Geometry check sheet. Reference: the model listing, model coordinates, mm. Face numbers are marked on the shaded views. A direction names the side the tool comes from. Coordinates: 2 decimals unless noted, no trailing zeros. Write each loop counter-clockwise with the first axis right and the second up, starting at its lowest first coordinate (ties: lowest second). Pieces come first, ordered by that corner, then holes.
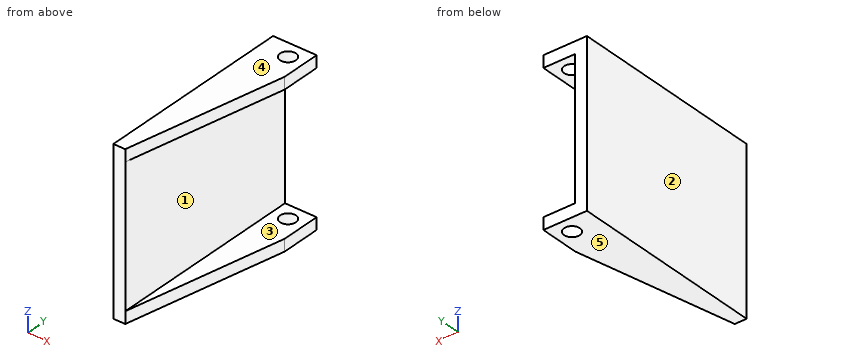
from build123d import *

# Parameters (mm, degrees)
SKETCH1_W           = 40.99099099
SKETCH1_H           = 50
BOSS_EXTRUDE1_DEPTH = 3
BOSS_EXTRUDE3_DEPTH = 3
SKETCH4_R           = 2
CUT_EXTRUDE1_DEPTH  = 3


with BuildPart() as part:
    # Sketch1 → Boss-Extrude1 (new body)
    with BuildSketch(Plane(origin=(0, 0, 0), x_dir=(0, 0, -1), z_dir=(1, 0, 0))):
        Rectangle(SKETCH1_W, SKETCH1_H)
    extrude(amount=BOSS_EXTRUDE1_DEPTH)

    # Sketch3 → Boss-Extrude3 (add)
    with BuildSketch(Plane.XY.offset(20.495495495)):
        Polygon((3, 25), (11, 25), (11, 15), (3, -25), align=None)
    boss_extrude3 = extrude(amount=-BOSS_EXTRUDE3_DEPTH)

    # Sketch4 → Cut-Extrude1 (cut)
    with BuildSketch(Plane.XY.offset(20.495495495)):
        with Locations((7, 21)):
            Circle(SKETCH4_R)
    cut_extrude1 = extrude(amount=-CUT_EXTRUDE1_DEPTH, mode=Mode.SUBTRACT)

    # Mirror1: Boss-Extrude3, Cut-Extrude1 across plane
    add(boss_extrude3.mirror(Plane.XY))
    add(cut_extrude1.mirror(Plane.XY), mode=Mode.SUBTRACT)


solid = part.part
1. Sectioned sample at D-D, the plane x = 10.25. Record the boundary of the cut face in (y, z), and give its area (3 significant figures).
Computed values:
outline: (11.25, -20.5) - (25, -20.5) - (25, -17.5) - (11.25, -17.5) - close; (11.25, 17.5) - (25, 17.5) - (25, 20.5) - (11.25, 20.5) - close
area: 82.5 mm2
2. Draft check along Z on the marked faces 3, 4 and 5. Enter one of: released by +Z, released by -Z, zero draft, split by the parting line, or undercut.
Computed values:
face 3: undercut
face 4: released by +Z
face 5: released by -Z
3. Thickness scan on line 1 along Z through (x, y) = (3.25, 15.5); line 2 along X through (y, z) = (-15, -10.5); line 3 along X through (y, z) = (11, 18.5). Record the ranges inside material, lowest first.
Computed values:
line 1: z = -20.5 to -17.5, 17.5 to 20.5
line 2: x = 0 to 3
line 3: x = 0 to 10.2
4. Gauge pin test, flat ends, axial feed: pin 1 Ø8 at (y, z) = (1.5, 13) entering from +X; pin 2 Ø1 at (x, z) = (9, -16) entering from +Y; pin 3 Ø6.5 at (x, y) = (9, 0) entering from +Z. Record the tip position at first contact, or that the pin passes through.
Computed values:
pin 1: stops at x = 3
pin 2: passes through
pin 3: stops at z = 20.5
5. Sectioned sample at B-B, the plane y = 21. Record the boundary of the cut face in (x, z), and give its area (3 significant figures).
Computed values:
outline: (0, -20.5) - (5, -20.5) - (5, -17.5) - (3, -17.5) - (3, 17.5) - (5, 17.5) - (5, 20.5) - (0, 20.5) - close; (9, -20.5) - (11, -20.5) - (11, -17.5) - (9, -17.5) - close; (9, 17.5) - (11, 17.5) - (11, 20.5) - (9, 20.5) - close
area: 147 mm2
6. Sectioned sample at C-C, the plane y = -3. Record the boundary of the cut face in (x, z), and give its area (3 significant figures).
Computed values:
outline: (0, -20.5) - (7.4, -20.5) - (7.4, -17.5) - (3, -17.5) - (3, 17.5) - (7.4, 17.5) - (7.4, 20.5) - (0, 20.5) - close
area: 149 mm2
7. Access from +Z, -Z, +X, -X, +Y, -Y to the whole of each face (thin tool, end or side, straight path). Record for the marked faces 1 and 2.
Computed values:
face 1: +X, +Y, -Y
face 2: +Z, -Z, -X, +Y, -Y
8. Sectioned sample at A-A, the plane x = 7. Record the boundary of the cut face in (y, z).
Computed values:
outline: (-5, -20.5) - (19, -20.5) - (19, -17.5) - (-5, -17.5) - close; (-5, 17.5) - (19, 17.5) - (19, 20.5) - (-5, 20.5) - close; (23, -20.5) - (25, -20.5) - (25, -17.5) - (23, -17.5) - close; (23, 17.5) - (25, 17.5) - (25, 20.5) - (23, 20.5) - close
